The drawing under review shows one solid part. Ordinate dimensions are in mm from its lowest x, y, z. A direction names the side the tool comes from. Coordinates: 2 decimals unless noted, no trailing zeros. Loops run counter-clockwise (first coordinate to the right, second up) from the corner with the lowest first, then second, coordinate; pieces in that order, holes last. Notation, with made-up numbers: M 0.5,4 L 30.5,4 A33 cw 30.5,32 Z; hole C 81.5,75.25 d5. An arc over 180 degrees is marked long. Answer as a JSON object with one key per item and string values. Group by question number.
1. Consider section C-C (y = 21). State the section outline as (x, z) points, then the cut area to 3 significant figures.
2. Consider section A-A (z = 47.5). State the section outline as (x, y) points, then the cut area to 3 significant figures.
3. Machinability: for the marked faces 1 and 2, which of the approach directions +Z, -Z, +X, -X, +Y, -Y give a long, thin tool a straight path to every point of the face, cutting with its end or side? Answer none if there is none.
4. To check wall thickness, follow probe 1 along Y at (x, z) = (38, 66); probe 2 along Z at (x, y) = (40.95, 21). State the ranges of each line that lie inside material, in increasing order.
5. Draft analysis for pull direction Y (two halves, no side actions). For the marked faces 3, 4 and 5, state which applies: +Y half, -Y half, draft (parallel to the pull), parting line (faces both ways), or undercut.
6. Insertion check: pin 1 (1 mm diameter, centred on x = 22, y = 36.5, fed in from -Z). The pin has a flat end and moves straight along its axis. Give the tip position at first contact, or say it passes through.
7. Consider section D-D (z = 18). State the section outline as (x, y) points.
8. Consider section B-B (x = 21). State the section outline as (y, z) points.
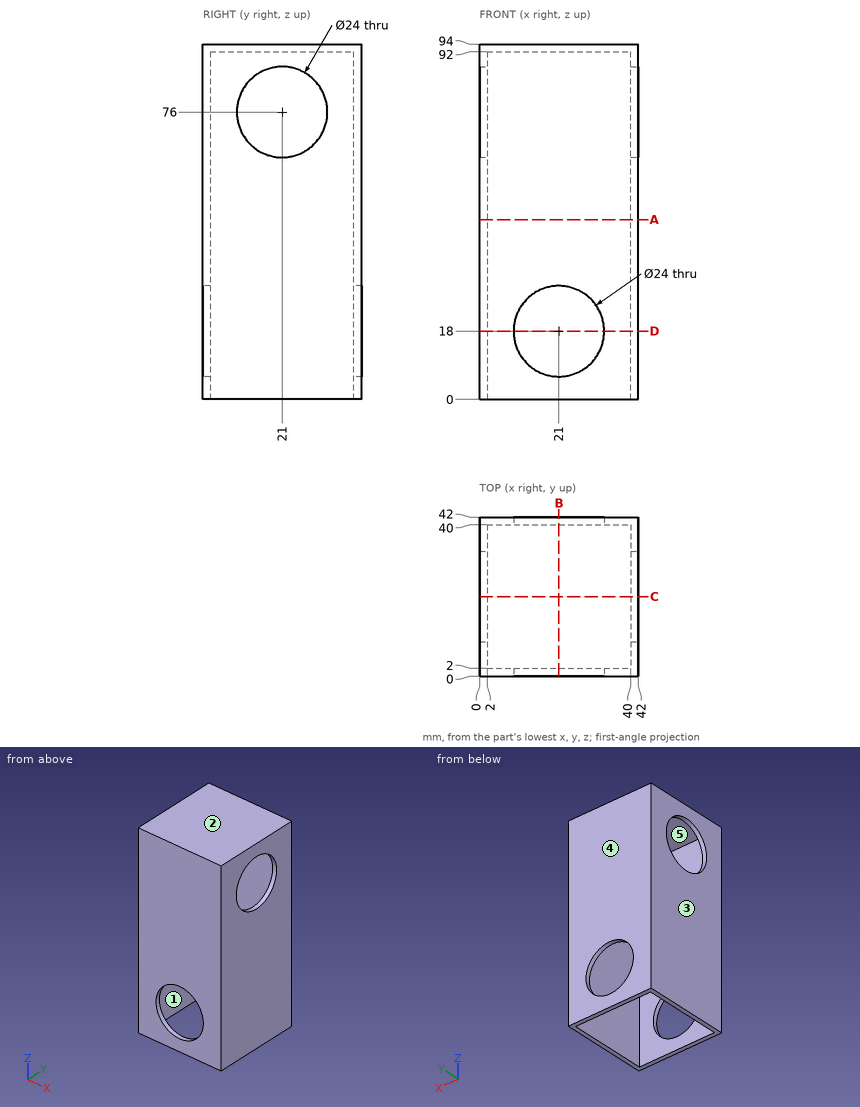
Findings below:
{
 "1": {"outline": "M 0,0 L 2,0 L 2,64 L 0,64 Z; M 0,88 L 2,88 L 2,92 L 40,92 L 40,88 L 42,88 L 42,94 L 0,94 Z; M 40,0 L 42,0 L 42,64 L 40,64 Z", "area": "356 mm^2"},
 "2": {"outline": "M 0,0 L 42,0 L 42,42 L 0,42 Z; hole M 2,2 L 40,2 L 40,40 L 2,40 Z", "area": "320 mm^2"},
 "3": {"face 1": "-Z", "face 2": "+Z, +X, -X, +Y, -Y"},
 "4": {"probe 1": "y = 0 to 2, 40 to 42", "probe 2": "z = 0 to 64, 88 to 94"},
 "5": {"face 3": "draft", "face 4": "+Y half", "face 5": "undercut"},
 "6": {"pin 1": "stops at z = 92"},
 "7": {"outline": "M 0,0 L 9,0 L 9,2 L 2,2 L 2,40 L 9,40 L 9,42 L 0,42 Z; M 33,0 L 42,0 L 42,42 L 33,42 L 33,40 L 40,40 L 40,2 L 33,2 Z"},
 "8": {"outline": "M 0,0 L 2,0 L 2,6 L 0,6 Z; M 0,30 L 2,30 L 2,92 L 40,92 L 40,30 L 42,30 L 42,94 L 0,94 Z; M 40,0 L 42,0 L 42,6 L 40,6 Z"}
}
